from build123d import *

# Parameters (mm, degrees)
BOSS_EXTRUDE1_DEPTH               = 3.175
F_6_CLEARANCE_HOLE1_D             = 4.3053
F_4_CLEARANCE_HOLE1_D             = 3.4544
F_6_CLEARANCE_HOLE2_D             = 4.3053
F_3_8_0_375_DIAMETER_HOLE1_D      = 9.525
F_1_2_0_5_DIAMETER_HOLE1_D        = 12.7
OBOGS_ROTARY_ANTI_ROTATION_HOLE_D = 3.81


with BuildPart() as part:
    # Sketch1 → Boss-Extrude1 (new body)
    with BuildSketch(Plane.XY):
        Polygon((112.268, 0), (0, 0), (0, -148.336), (112.268, -138.684), align=None)
    extrude(amount=-BOSS_EXTRUDE1_DEPTH)

    # #6 Clearance Hole1 (through all)
    with Locations(Plane.XY):
        with Locations((6.731, -133.35), (107.3785, -128.5875), (107.3785, -66.675), (4.8895, -76.2)):
            Hole(F_6_CLEARANCE_HOLE1_D / 2)

    # #4 Clearance Hole1 (through all)
    with Locations(Plane.XY):
        with Locations((18.644469576, -70.03220158), (57.60279842, -62.459469576), (65.175530424, -101.41779842), (26.21720158, -108.990530424), (65.891864398, -135.837535562), (88.720535562, -134.641135602), (87.524135602, -111.812464438), (64.695464438, -113.008864398)):
            Hole(F_4_CLEARANCE_HOLE1_D / 2)

    # #6 Clearance Hole2 (through all)
    with Locations(Plane.XY):
        with Locations((36.322, -16.51), (85.6615, -47.625)):
            Hole(F_6_CLEARANCE_HOLE2_D / 2)

    # 3/8 (0.375) Diameter Hole1 (through all)
    with Locations(Plane.XY):
        with Locations((76.2, -25.4)):
            Hole(F_3_8_0_375_DIAMETER_HOLE1_D / 2)

    # 1/2 (0.5) Diameter Hole1 (through all)
    with Locations(Plane.XY):
        with Locations((17.526, -22.352)):
            Hole(F_1_2_0_5_DIAMETER_HOLE1_D / 2)

    # OBOGS Rotary Anti Rotation Hole (through all)
    with Locations(Plane(origin=(0, 0, -3.175), x_dir=(-1, 0, 0), z_dir=(0, 0, -1))):
        with Locations((-66.792027829, -25.458354734)):
            Hole(OBOGS_ROTARY_ANTI_ROTATION_HOLE_D / 2)


solid = part.part
Geometry check sheet. Reference: the model listing, model coordinates, mm. Give positions to 0.01 mm unless a question says otherwise; leave off trailing zeros. Order: outer loops, then holes, each group sorted by start corner. A loop starts at its lowest first (then second) coordinate and runs counter-clockwise, first axis right, second up. Notation, with made-up numbers: M 82.5,67.25 L 107.5,67.25 A18 ccw 107.5,93.25 Z; hole C 62,69 d8. An arc over 180 degrees is marked long. Use a Markdown table: item, result.
Item 1: Material ranges on line 1 along X through (y, z) = (-23.5, -2); line 2 along X through (y, z) = (-46, -1.95); line 3 along X through (y, z) = (-61.5, -2.65), recorded low to high.
Answers follow:
| item | result |
|---|---|
| line 1 | x = 0 to 11.28, 23.77 to 71.83, 80.57 to 112.27 |
| line 2 | x = 0 to 84.25, 87.07 to 112.27 |
| line 3 | x = 0 to 56.17, 59.04 to 112.27 |
Item 2: Section check C-C (x = 93.5). Record the cut outline in (y, z) (3 decimals), and give its area (3 significant figures).
Answers follow:
| item | result |
|---|---|
| outline | M -140.298,-3.175 L 0,-3.175 L 0,0 L -140.298,0 Z |
| area | 445 mm2 |
Item 3: Section check D-D (x = 52.5). Record the cut outline in (y, z) (3 decimals).
Answers follow:
| item | result |
|---|---|
| outline | M -143.822,-3.175 L 0,-3.175 L 0,0 L -143.822,0 Z |
Item 4: Section check A-A (y = -76.2). Record the cut outline in (x, z) (3 decimals), and give its area (3 significant figures).
Answers follow:
| item | result |
|---|---|
| outline | M 0,-3.175 L 2.737,-3.175 L 2.737,0 L 0,0 Z; M 7.042,-3.175 L 112.268,-3.175 L 112.268,0 L 7.042,0 Z |
| area | 343 mm2 |
Item 5: Section check B-B (z = -1.9). State how many separate pieces and enclosed holes the cut face has, and give its area (3 significant figures).
Answers follow:
| item | result |
|---|---|
| separate pieces | 1 |
| enclosed holes | 17 |
| area | 15,700 mm2 |
Item 6: Draft check along X on faces 1 (the flat face through (0, -73, -2)), 2 (the cylindrical face through (65.4, -99.705, -1.61)), 3 (the flat face through (55.348, -143.578, -1.565)). Enter one of: +X half, -X half, draft (parallel to the pull), parting line (faces both ways), or undercut.
Answers follow:
| item | result |
|---|---|
| face 1 | -X half |
| face 2 | undercut |
| face 3 | +X half |
Item 7: Depth check by flat-ended pin: P1, Ø3, axis at x = 57.6, y = -62.46, coming from the +Z side. Enter the tip coordinate at first touch or a pass-through.
Answers follow:
| item | result |
|---|---|
| P1 | passes through |
